Design review of the part built by this model. Coordinates are the model's own, in mm. A direction names the side the tool comes from. Give positions to 0.01 mm unless a question says otherwise; leave off trailing zeros. Loops run counter-clockwise (first coordinate to the right, second up) from the corner with the lowest first, then second, coordinate; pieces in that order, holes last.
from build123d import *

# Parameters (mm, degrees)
BASE_FLANGE1_DEPTH = 76.2
CUT_EXTRUDE1_DEPTH = 117.26744224
SKETCH7_R          = 3.3782
CUT_EXTRUDE2_DEPTH = 117.26744224
FILLET1_R          = 3.175


# Sheet-metal steps are written as plain solids
with BuildPart() as part:
    # Sketch1 → Base-Flange1 (new body)
    with BuildSketch(Plane.XY):
        with BuildLine():
            Line((85.725, 19.05), (85.725, 6.35))
            ThreePointArc((85.725, 6.35), (83.865128061, 1.859871939), (79.375, 0))
            Line((79.375, 0), (6.35, 0))
            ThreePointArc((6.35, 0), (1.859871939, 1.859871939), (0, 6.35))
            Line((0, 6.35), (0, 19.05))
            Line((0, 19.05), (3.175, 19.05))
            Line((3.175, 19.05), (3.175, 6.35))
            ThreePointArc((3.175, 6.35), (4.10493597, 4.10493597), (6.35, 3.175))
            Line((6.35, 3.175), (79.375, 3.175))
            ThreePointArc((79.375, 3.175), (81.62006403, 4.10493597), (82.55, 6.35))
            Line((82.55, 6.35), (82.55, 19.05))
            Line((82.55, 19.05), (85.725, 19.05))
        make_face()
    extrude(amount=BASE_FLANGE1_DEPTH)

    # Sketch6 → Cut-Extrude1 (cut, through all)
    with BuildSketch(Plane.ZY):
        with BuildLine():
            Line((35.6108, 11.1125), (35.6108, 14.2875))
            ThreePointArc((35.6108, 14.2875), (38.1, 16.7767), (40.5892, 14.2875))
            Line((40.5892, 14.2875), (40.5892, 11.1125))
            ThreePointArc((40.5892, 11.1125), (38.1, 8.6233), (35.6108, 11.1125))
        make_face()
        with BuildLine():
            Line((10.2108, 11.1125), (10.2108, 14.2875))
            ThreePointArc((10.2108, 14.2875), (12.7, 16.7767), (15.1892, 14.2875))
            Line((15.1892, 14.2875), (15.1892, 11.1125))
            ThreePointArc((15.1892, 11.1125), (12.7, 8.6233), (10.2108, 11.1125))
        make_face()
        with BuildLine():
            Line((61.0108, 11.1125), (61.0108, 14.2875))
            ThreePointArc((61.0108, 14.2875), (63.5, 16.7767), (65.9892, 14.2875))
            Line((65.9892, 14.2875), (65.9892, 11.1125))
            ThreePointArc((65.9892, 11.1125), (63.5, 8.6233), (61.0108, 11.1125))
        make_face()
    extrude(amount=-CUT_EXTRUDE1_DEPTH, mode=Mode.SUBTRACT)

    # Sketch7 → Cut-Extrude2 (cut, through all)
    with BuildSketch(Plane.XZ):
        with Locations(Location((61.9125, 38.1, 0), (0, 0, 270))):
            Circle(SKETCH7_R)
        with Locations(Location((23.8125, 38.1, 0), (0, 0, 270))):
            Circle(SKETCH7_R)
    extrude(amount=-CUT_EXTRUDE2_DEPTH, mode=Mode.SUBTRACT)

    # Fillet1
    fillet1_edges = [part.edges().sort_by_distance(p)[0] for p in [
        (1.5875, 19.05, 0),
        (84.1375, 19.05, 0),
        (1.5875, 19.05, 76.2),
        (84.1375, 19.05, 76.2),
    ]]
    fillet(fillet1_edges, radius=FILLET1_R)


solid = part.part
Q1. Wall thickness on line 1 (X direction, y = 13, z = 52.5) (3 decimals); line 2 (X direction, y = 0.8, z = 38.1); line 3 (X direction, y = 1.6, z = 38.1): over which ranges is each line inside the solid? List them lowest first.
Results:
line 1: x = 0 to 3.175, 82.55 to 85.725
line 2: x = 3.26 to 20.43, 27.19 to 58.53, 65.29 to 82.46
line 3: x = 2.14 to 20.43, 27.19 to 58.53, 65.29 to 83.59
Q2. Take a section at B-B (z = 38.1). Give the boundary of the cut face in (x, y) (3 decimals), plus the area to 3 significant figures.
Results:
outline: (0, 6.35) arc R6.35 ccw to (6.35, 0) - (20.434, 0) - (20.434, 3.175) - (6.35, 3.175) arc R3.175 cw to (3.175, 6.35) - (3.175, 8.623) - (0, 8.623) - close; (0, 16.777) - (3.175, 16.777) - (3.175, 19.05) - (0, 19.05) - close; (27.191, 0) - (58.534, 0) - (58.534, 3.175) - (27.191, 3.175) - close; (65.291, 0) - (79.375, 0) arc R6.35 ccw to (85.725, 6.35) - (85.725, 8.623) - (82.55, 8.623) - (82.55, 6.35) arc R3.175 cw to (79.375, 3.175) - (65.291, 3.175) - close; (82.55, 16.777) - (85.725, 16.777) - (85.725, 19.05) - (82.55, 19.05) - close
area: 265 mm2
Q3. Take a section at C-C (x = 25). Give the boundary of the cut face in (y, z) (3 decimals).
Results:
outline: (0, 0) - (3.175, 0) - (3.175, 34.937) - (0, 34.937) - close; (0, 41.263) - (3.175, 41.263) - (3.175, 76.2) - (0, 76.2) - close
Q4. Draft analysis for pull direction X (two halves, no side actions). For faces 1 (the face through (1.565, 8.624, 38.155)), 2 (the face through (1.91, 1.81, 37.57)), 3 (the face through (84, 2, 38)), 4 (the face through (23.961, 1.565, 41.475)), state which applies: pulls with the +X half, pulls with the -X half, needs draft (parallel to the pull), parting line crosses it, or undercut.
Results:
face 1: needs draft
face 2: pulls with the -X half
face 3: pulls with the +X half
face 4: undercut
Q5. Take a section at D-D (z = 67). Give the boundary of the cut face in (x, y) (3 decimals), plus the area to 3 significant figures.
Results:
outline: (0, 6.35) arc R6.35 ccw to (6.35, 0) - (79.375, 0) arc R6.35 ccw to (85.725, 6.35) - (85.725, 19.05) - (82.55, 19.05) - (82.55, 6.35) arc R3.175 cw to (79.375, 3.175) - (6.35, 3.175) arc R3.175 cw to (3.175, 6.35) - (3.175, 19.05) - (0, 19.05) - close
area: 360 mm2
Q6. Tool access review of faces 5 (the face through (42, 3.175, 38)), 6 (the face through (84, 13, 35.611)), 7 (the face through (85.725, 17, 38)): name each direction out of +Z, -Z, +X, -X, +Y, -Y from which nothing blocks a thin tool from reaching the whole face with its end or side.
Results:
face 5: +Z, -Z, +Y
face 6: +X, -X
face 7: +Z, -Z, +X, +Y, -Y
Q7. Take a section at A-A (z = 12.7). Give the boundary of the cut face in (x, y) (3 decimals), plus the area to 3 significant figures.
Results:
outline: (0, 6.35) arc R6.35 ccw to (6.35, 0) - (79.375, 0) arc R6.35 ccw to (85.725, 6.35) - (85.725, 8.623) - (82.55, 8.623) - (82.55, 6.35) arc R3.175 cw to (79.375, 3.175) - (6.35, 3.175) arc R3.175 cw to (3.175, 6.35) - (3.175, 8.623) - (0, 8.623) - close; (0, 16.777) - (3.175, 16.777) - (3.175, 19.05) - (0, 19.05) - close; (82.55, 16.777) - (85.725, 16.777) - (85.725, 19.05) - (82.55, 19.05) - close
area: 308 mm2
Q8. Insertion check: pin 1 (3 mm diameter, centred on x = 28, z = 13, fed in from +Y) (3 decimals); pin 2 (5.5 mm diameter, centred on x = 23.81, z = 38.1, fed in from +Y). Each pin has a flat end and moves straight along its axis. Give the tip position at first contact, or say it passes through.
Results:
pin 1: stops at y = 3.175
pin 2: passes through
